Design review of the part built by this model. Coordinates are the model's own, in mm. A direction names the side the tool comes from. Coordinates: 2 decimals unless noted, no trailing zeros. Write each loop counter-clockwise with the first axis right and the second up, starting at its lowest first coordinate (ties: lowest second). Pieces come first, ordered by that corner, then holes.
Q1. Take a section at B-B, the plane z = 2.2. State how many separate pieces and enclosed holes the cut face has, plus the area to 3 significant figures.
Q2. Take a section at A-A, the plane x = 12.7. Write out the cut boundary in (y, z) (3 decimals), plus the area to 3 significant figures.
Q3. For L1, parallel to X at y = 39, z = 1.4; L2, parallel to Y at x = 12.7, z = 1.1; L3, parallel to Y at x = 134, z = 0.7, list the stretches that pass through material, from the lowest coordinate up.
Q4. For pin 1 Ø7.5 at (x, y) = (130.19, -66.89) entering from +Z (3 decimals); pin 2 Ø1.5 at (y, z) = (23.5, 1) entering from +X; pin 3 Ø6 at (x, y) = (125.28, -117.21) entering from +Z; pin 4 Ø1 at (y, z) = (-0.5, 1) entering from -X, all flat-tipped, find the tip position at first contact; note any pin that passes through.
Q5. For faces 1 (the flat face through (168.73, -138.61, 1.57)), 2 (the cylindrical face through (35.187, 43.459, 1.565)), list the 3-axis set-ups (+Z, -Z, +X, -X, +Y, -Y) from which the entire face can be reached by the end or side of a thin tool; tool diameter is ignored.
Q6. The part is to be moulded in two halves that separate along X. For faces 3 (the cylindrical face through (122.663, -115.205, 1.565)), 4 (the cylindrical face through (136.86, -16.7, 1.57)), 5 (the cylindrical face through (114.272, -77.079, 1.565)), 6 (the flat face through (124.9, -208.89, 1.57)), say which applies: released by +X, released by -X, zero draft, split by the parting line, or undercut.
Autodesk Inventor part; units mm, degrees
ref_plane "YZ Plane" through (0, 0, 0) normal (1, 0, 0) x (0, 1, 0)
ref_plane "XZ Plane" through (0, 0, 0) normal (0, 1, 0) x (-1, 0, 0)
ref_plane "XY Plane" through (0, 0, 0) normal (0, 0, 1) x (1, 0, 0)
sketch "Sketch1" plane through (0, 0, 0) normal (0, 0, 1) x (1, 0, 0)
  circle A0 centre (146.7716, -66.8928) radius 3.302
  circle A1 centre (142.4086, -41.8704) radius 3.302
  circle A2 centre (115.6509, -18.469) radius 3.302
  circle A3 centre (12.7, 67.1787) radius 3.302
  circle A4 centre (37.7225, 62.8157) radius 3.302
  circle A5 centre (61.6236, 54.2194) radius 3.302
  circle A6 centre (-37.6212, 45.6905) radius 3.302
  circle A7 centre (-12.7, 67.1787) radius 3.302
  circle A8 centre (-61.6236, 54.2194) radius 3.302
  circle A9 centre (-133.8122, -17.9693) radius 3.302
  circle A10 centre (-130.192, -66.8928) radius 3.302
  circle A11 centre (-146.7716, -66.8928) radius 3.302
  circle A12 centre (-142.4086, -41.8704) radius 3.302
  circle A13 centre (-125.2833, -41.9717) radius 3.302
  circle A14 centre (-115.6509, -18.469) radius 3.302
  circle A15 centre (-37.7225, 62.8157) radius 3.302
  circle A16 centre (-12.7, 50.5992) radius 3.302
  circle A17 centre (-61.1239, 36.0581) radius 3.302
  circle A18 centre (61.1239, 36.0581) radius 3.302
  circle A19 centre (37.6212, 45.6905) radius 3.302
  circle A20 centre (12.7, 50.5992) radius 3.302
  circle A21 centre (133.8122, -17.9693) radius 3.302
  circle A22 centre (125.2833, -41.9717) radius 3.302
  circle A23 centre (130.192, -66.8928) radius 3.302
  arc A24 (165.1, -79.5928) -> (-165.1, -79.5928) centre (0, -79.5928) ccw
  line L0 (-114.3, -79.5928) -> (-165.1, -79.5928)
  arc A25 (114.3, -79.5928) -> (-114.3, -79.5928) centre (0, -79.5928) ccw
  line L1 (165.1, -79.5928) -> (114.3, -79.5928)
  circle A26 centre (-146.7716, -92.2928) radius 3.302
  circle A27 centre (-142.4086, -117.3153) radius 3.302
  circle A28 centre (-115.6509, -140.7167) radius 3.302
  circle A29 centre (-12.7, -226.3644) radius 3.302
  circle A30 centre (-37.7225, -222.0014) radius 3.302
  circle A31 centre (-61.6236, -213.4051) radius 3.302
  circle A32 centre (37.6212, -204.8761) radius 3.302
  circle A33 centre (12.7, -226.3644) radius 3.302
  circle A34 centre (61.6236, -213.4051) radius 3.302
  circle A35 centre (133.8122, -141.2164) radius 3.302
  circle A36 centre (130.192, -92.2928) radius 3.302
  circle A37 centre (146.7716, -92.2928) radius 3.302
  circle A38 centre (142.4086, -117.3153) radius 3.302
  circle A39 centre (125.2833, -117.214) radius 3.302
  circle A40 centre (115.6509, -140.7167) radius 3.302
  circle A41 centre (37.7225, -222.0014) radius 3.302
  circle A42 centre (12.7, -209.7849) radius 3.302
  circle A43 centre (61.1239, -195.2437) radius 3.302
  circle A44 centre (-61.1239, -195.2437) radius 3.302
  circle A45 centre (-37.6212, -204.8761) radius 3.302
  circle A46 centre (-12.7, -209.7849) radius 3.302
  circle A47 centre (-133.8122, -141.2164) radius 3.302
  circle A48 centre (-125.2833, -117.214) radius 3.302
  circle A49 centre (-130.192, -92.2928) radius 3.302
  arc A50 (-165.1, -79.5928) -> (165.1, -79.5928) centre (0, -79.5928) ccw
  line L2 (114.3, -79.5928) -> (165.1, -79.5928)
  arc A51 (-114.3, -79.5928) -> (114.3, -79.5928) centre (0, -79.5928) ccw
  line L3 (-165.1, -79.5928) -> (-114.3, -79.5928)
  arc A52 (0, -257.3928) -> (0, 98.2072) centre (0, -79.5928) ccw
  line L4 (0, 98.2072) -> (0, 34.7072)
  line L5 (0, -193.8928) -> (0, -257.3928)
  point P0 (0, 0)
  dimension "d0" = 355.6
extrude "Extrusion1" add sketch "Sketch1" along normal blind 3.175 contours L1 A25 L4 A24 | A50 L5 A51 L1 | A24 L4 A52 L5 A50
sketch "Sketch2" plane through (0, 0, 0) normal (0, 0, -1) x (-1, 0, 0)
  arc A0 (0, 98.2072) -> (0, -257.3928) centre (0, -79.5928) ccw
  line L0 (-215.9, -184.3678) -> (-163.2323, -184.3678)
  line L1 (-152.4, -184.3678) -> (0, -184.3678)
  line L2 (152.4, -190.7178) -> (-152.4, -190.7178)
  line L3 (152.4, -190.7178) -> (-152.4, -190.7178)
  line L4 (-215.9, -181.1928) -> (-163.2323, -181.1928)
  line L5 (0, -190.7178) -> (-203.2, -190.7178)
  line L6 (-46.5518, -181.1928) -> (46.5518, -181.1928)
  line L7 (152.4, -181.1928) -> (-152.4, -181.1928)
  line L8 (-163.2323, -193.8928) -> (-215.9, -193.8928)
  line L9 (0, -184.3678) -> (-203.2, -184.3678)
  line L10 (-127, -193.8928) -> (-163.2323, -193.8928)
  arc A1 (0, 98.2072) -> (0, -257.3928) centre (0, -79.5928) ccw
  line L11 (-145.9119, -181.1928) -> (-145.9119, -193.8928)
  line L12 (-145.9119, -193.8928) -> (-136.1923, -193.8928)
  arc A2 (-145.9119, -181.1928) -> (-136.1923, -193.8928) centre (0, -79.5928) ccw
  line L13 (-145.9119, -181.1928) -> (-158.6119, -181.1928)
  line L14 (-158.6119, -181.1928) -> (-172.9857, -120.6879)
  line L15 (-145.9119, -193.8928) -> (-103.2908, -224.3128)
  arc A3 (-172.9857, -120.6879) -> (-145.9119, -181.1928) centre (0, -79.5928) ccw
  arc A4 (-145.9119, -181.1928) -> (-103.2908, -224.3128) centre (0, -79.5928) ccw
  line L16 (0, -79.5928) -> (-43.5104, -79.5928) construction
  line L17 (-145.9119, 22.0072) -> (-145.9119, 34.7072)
  line L18 (-145.9119, 22.0072) -> (-158.6119, 22.0072)
  line L19 (-158.6119, 22.0072) -> (-172.9857, -38.4978)
  line L20 (-145.9119, 34.7072) -> (-103.2908, 65.1271)
  arc A5 (-145.9119, 22.0072) -> (-172.9857, -38.4978) centre (0, -79.5928) ccw
  arc A6 (-103.2908, 65.1271) -> (-145.9119, 22.0072) centre (0, -79.5928) ccw
  point P0 (0, 0)
  dimension "d3" = 12.7
extrude "Extrusion3" add sketch "Sketch2" against normal blind 3.175
sketch "Sketch3" plane through (0, 0, 0) normal (0, 0, -1) x (-1, 0, 0)
  circle A0 centre (-61.1239, -195.2437) radius 3.302
  circle A1 centre (-12.7, -209.7849) radius 3.302
  circle A2 centre (-37.7225, -222.0014) radius 3.302
  circle A3 centre (-115.6509, -140.7167) radius 3.302
  circle A4 centre (-125.2833, -117.214) radius 3.302
  circle A5 centre (-142.4086, -117.3153) radius 3.302
  circle A6 centre (-146.7716, -92.2928) radius 3.302
  circle A7 centre (-130.192, -92.2928) radius 3.302
  circle A8 centre (-133.8122, -141.2164) radius 3.302
  circle A9 centre (-61.6236, -213.4051) radius 3.302
  circle A10 centre (-12.7, -226.3644) radius 3.302
  circle A11 centre (-37.6212, -204.8761) radius 3.302
  circle A12 centre (-130.192, -66.8928) radius 3.302
  circle A13 centre (-125.2833, -41.9717) radius 3.302
  circle A14 centre (-133.8122, -17.9693) radius 3.302
  circle A15 centre (-12.7, 50.5992) radius 3.302
  circle A16 centre (-37.6212, 45.6905) radius 3.302
  circle A17 centre (-61.1239, 36.0581) radius 3.302
  circle A18 centre (-61.6236, 54.2194) radius 3.302
  circle A19 centre (-37.7225, 62.8157) radius 3.302
  circle A20 centre (-12.7, 67.1787) radius 3.302
  circle A21 centre (-115.6509, -18.469) radius 3.302
  circle A22 centre (-142.4086, -41.8704) radius 3.302
  circle A23 centre (-146.7716, -66.8928) radius 3.302
  arc A24 (0, 34.7072) -> (0, -193.8928) centre (0, -79.5928) ccw
  line L0 (0, 98.2072) -> (0, 34.7072)
  arc A25 (0, 98.2072) -> (-103.2908, 65.1271) centre (0, -79.5928) ccw
  line L1 (-103.2908, 65.1271) -> (-145.9119, 34.7072)
  line L2 (-145.9119, 34.7072) -> (-145.9119, 22.0072)
  line L3 (-145.9119, 22.0072) -> (-158.6119, 22.0072)
  line L4 (-158.6119, 22.0072) -> (-172.9857, -38.4978)
  arc A26 (-172.9857, -38.4978) -> (-172.9857, -120.6879) centre (0, -79.5928) ccw
  line L5 (-172.9857, -120.6879) -> (-158.6119, -181.1928)
  line L6 (-158.6119, -181.1928) -> (-145.9119, -181.1928)
  line L7 (-145.9119, -181.1928) -> (-145.9119, -193.8928)
  line L8 (-145.9119, -193.8928) -> (-103.2908, -224.3128)
  arc A27 (-103.2908, -224.3128) -> (0, -257.3928) centre (0, -79.5928) ccw
  line L9 (0, -193.8928) -> (0, -257.3928)
  line L10 (-145.9119, -181.1928) -> (-158.6119, -181.1928)
  line L11 (-158.6119, -181.1928) -> (-178.9319, -181.1928)
  circle A28 centre (0, -79.5928) radius 177.8
  arc A29 (-172.4957, -170.8784) -> (-178.9319, -181.1928) centre (-169.0032, -180.223) ccw
  arc A30 (-172.4957, -170.8784) -> (-164.5857, -156.0467) centre (-176.9418, -158.9821) ccw
  arc A31 (-172.9857, -38.4978) -> (-172.9857, -120.6879) centre (0, -79.5928) ccw
  line L12 (0, -79.5928) -> (-220.3249, -79.5928)
  line L13 (-158.6119, -181.1928) -> (-172.9857, -120.6879)
  line L14 (-164.5857, -156.0467) -> (-158.6119, -181.1928)
  line L15 (-172.9857, -38.4978) -> (-164.5857, -3.139)
  line L16 (-158.6119, 22.0072) -> (-178.9319, 22.0072)
  arc A32 (-178.9319, 22.0072) -> (-172.4957, 11.6927) centre (-169.0032, 21.0374) ccw
  arc A33 (-164.5857, -3.139) -> (-172.4957, 11.6927) centre (-176.9418, -0.2036) ccw
  line L17 (-164.5857, -3.139) -> (-158.6119, 22.0072)
  point P0 (0, 0)
  point P1 (-159.6945, -176.6356)
  dimension "d8" = 20.32
  dimension "d9" = 12.7
extrude "Extrusion4" add sketch "Sketch3" against normal blind 3.175 contours A33 A32 L16 L4 | L5 L11 A29 A30
sketch "Sketch4" plane through (0, 0, 3.175) normal (0, 0, 1) x (1, 0, 0)
  circle A0 centre (96.1901, -201.0584) radius 3.302
  circle A1 centre (96.1901, 41.8727) radius 3.302
  point P0 (0, 0)
extrude "Extrusion5" cut sketch "Sketch4" against normal blind 3.175
properties part number "13in outer coil"
Responses:
1. separate pieces: 1
1. enclosed holes: 26
1. area: 29,500 mm2
2. outline: (-256.939, 0) - (-229.666, 0) - (-229.666, 3.175) - (-256.939, 3.175) - close; (-223.062, 0) - (-213.087, 0) - (-213.087, 3.175) - (-223.062, 3.175) - close; (-206.483, 0) - (-193.185, 0) - (-193.185, 3.175) - (-206.483, 3.175) - close; (33.999, 0) - (47.297, 0) - (47.297, 3.175) - (33.999, 3.175) - close; (53.901, 0) - (63.877, 0) - (63.877, 3.175) - (53.901, 3.175) - close; (70.481, 0) - (97.753, 0) - (97.753, 3.175) - (70.481, 3.175) - close
2. area: 321 mm2
3. L1: x = 0 to 59.62, 62.62 to 94.56, 97.82 to 139.9
3. L2: y = -256.94 to -229.67, -223.06 to -213.09, -206.48 to -193.19, 34 to 47.3, 53.9 to 63.88, 70.48 to 97.75
3. L3: y = -202.39 to -144.51, -137.92 to -21.27, -14.67 to 43.21
4. pin 1: stops at z = 3.175
4. pin 2: stops at x = 145.91
4. pin 3: passes through
4. pin 4: stops at x = 82.03
5. face 1: +Z, -Z, +X
5. face 2: +Z, -Z
6. face 3: undercut
6. face 4: undercut
6. face 5: released by -X
6. face 6: released by +X
